Read the model definition and answer for the solid it produces. Units are mm, in the model's axes. A direction names the side the tool comes from. Round coordinates to 2 decimals unless told otherwise and drop trailing zeros. Loops run counter-clockwise (first coordinate to the right, second up) from the corner with the lowest first, then second, coordinate; pieces in that order, holes last. Notation, with made-up numbers: M -30,-25.75 L 2,-25.75 A17 ccw 2,-4.75 Z; hole C 52.5,4.25 d5. An arc over 180 degrees is marked long. Write each question's results on one line, items separated by ' | '.
from build123d import *

# Parameters (mm, degrees)
F1_DEPTH = 5
F2_R     = 0.99999


# Not quite as in the source:
# - a fillet or chamfer is up to 0.001 mm smaller than in the source, because OpenCascade refuses the exact size
# - a feature names something its author has since deleted; it is built from what else it names


with BuildPart() as f1:
    # F0 (on Front) → F1 (new body)
    with BuildSketch(Plane.XZ):
        Polygon((-4, 0), (0, 0), (0, -2.4), (-2, -2.4), (-2, -3.4), (7, -3.4), (7, -2.4), (5, -2.4), (5, 0), (10, 0), (10, 8), (-4, 8), (-4, 6), (8, 6), (8, 2), (-4, 2), align=None)
    extrude(amount=F1_DEPTH)

    # F2 (radius 1 in the source; OpenCascade refuses exactly that, so slightly less here)
    f2_edges = [f1.edges().sort_by_distance(p)[0] for p in [
        (8, -2.5, 6),
        (8, -2.5, 2),
        (10, -2.5, 0),
        (10, -2.5, 8),
        (-4, -2.5, 8),
        (-4, -2.5, 6),
        (-4, -2.5, 0),
        (-4, -2.5, 2),
    ]]
    fillet(f2_edges, radius=F2_R)


solid = f1.part
Item 1: Flat-ended cylindrical pins translate along their axes: pin 1 (2.5 mm diameter, centred on y = -3, z = -1, fed in from +X); pin 2 (0.8 mm diameter, centred on y = -2.5, z = -3, fed in from +X); pin 3 (1.1 mm diameter, centred on y = -3, z = -3, fed in from -X). Find the tip coordinate at first contact, or state that the pin passes through.
Outcome:
pin 1: stops at x = 9.66 | pin 2: stops at x = 7 | pin 3: stops at x = -2
Item 2: The part is cut by section A-A (x = 0.25). Determine the outline of the cut face in (y, z).
Outcome:
outline: M -5,-3.4 L 0,-3.4 L 0,2 L -5,2 Z; M -5,6 L 0,6 L 0,8 L -5,8 Z
Item 3: The mould has two halves that part along Z. Classify faces 5 (the face through (9.699, -2.535, 0.285)), 6 (the face through (-1, -2, -2.4)), 7 (the face through (3, -5, 1)), 8 (the face through (9.715, -2.535, 7.699)): pulls with the +Z half, pulls with the -Z half, needs draft (parallel to the pull), parting line crosses it, or undercut.
Outcome:
face 5: pulls with the -Z half | face 6: undercut | face 7: needs draft | face 8: pulls with the +Z half
Item 4: Straight lines are drawn through the part: line 1 (Z direction, x = 0.75, y = -2.6); line 2 (Z direction, x = 6, y = -4.65); line 3 (X direction, y = -1.1, z = -1). For each, find the intervals that lie inside material, in ascending order.
Outcome:
line 1: z = -3.4 to 2, 6 to 8 | line 2: z = -3.4 to -2.4, 0 to 2, 6 to 8 | line 3: x = 0 to 5
Item 5: The part is cut by section D-D (z = -0.5). Determine the outline of the cut face in (x, y).
Outcome:
outline: M 0,-5 L 5,-5 L 5,0 L 0,0 Z
Item 6: The part is cut by section B-B (x = 6.5). Determine the outline of the cut face in (y, z), plus the area to 3 significant figures.
Outcome:
outline: M -5,-3.4 L 0,-3.4 L 0,-2.4 L -5,-2.4 Z; M -5,0 L 0,0 L 0,2 L -5,2 Z; M -5,6 L 0,6 L 0,8 L -5,8 Z | area: 25.0 mm2
Item 7: For faces 1 (the face through (6, -2, -2.4)), 2 (the face through (7, -2, -3)), 3 (the face through (7.715, -2.535, 2.301)), 4 (the face through (-2, -2, -3)), determine the directions among +Z, -Z, +X, -X, +Y, -Y from which every point of the face is accessible in a straight line to the end or side of a thin tool.
Outcome:
face 1: +X, +Y, -Y | face 2: -Z, +X, +Y, -Y | face 3: -X, +Y, -Y | face 4: -Z, -X, +Y, -Y
